Can you work these out from the model? Positions are in its coordinate system, mm. Round coordinates to 2 decimals unless told otherwise and drop trailing zeros. Write each loop counter-clockwise with the first axis right and the second up, starting at its lowest first coordinate (ties: lowest second). Pieces come first, ordered by that corner, then holes. Notation, with made-up numbers: M -18,-27.5 L 41,-27.5 A25 ccw 41,1.5 Z; hole C 66,34 d5. An arc over 180 degrees is marked long. Answer as a JSON object with one key per item and string values. Group by question number.
1) Suppose I cut it at A-A, the plane x = 40. Write out the boundary of the cut face in (y, z), and give its area (3 significant figures).
2) I'm going to push a flat-ended pin straight in: pin 1 Ø3.5 at (x, z) = (60, 0) entering from +Y. Where does the tip first touch, or does it pass through?
3) If we mould it in two halves opening along X, with no side actions, what happens to faces 1 (the flat face through (31, 1, 4)), 2 (the cylindrical face through (8.536, 1.521, -0.325)), 3 (the cylindrical face through (74, 1, 0))? For each: +X half, -X half, draft (parallel to the pull), parting line (faces both ways), or undercut.
4) Please list where these lines run through material, in increasing order: L1, parallel to Z at x = 70, y = 2.2; L2, parallel to Z at x = 10.5, y = 0.6; L3, parallel to X at y = 2.2, z = -3. Write a range as [from, to].
5) Suppose I cut it at B-B, the plane y = 0.8. State how many separate pieces and enclosed holes the cut face has, and give its area (3 significant figures).
from build123d import *

# Parameters (mm, degrees)
OUTER_BODY_DEPTH = 3
SKETCH8_R        = 1.5
HOLES_DEPTH      = 75.168726563


with BuildPart() as part:
    # Sketch1 → Outer Body (new body)
    with BuildSketch(Plane(origin=(0, 0, 0), x_dir=(1, 0, 0), z_dir=(0, 1, 0))):
        with BuildLine():
            Line((-10, 4), (70, 4))
            ThreePointArc((70, 4), (74, 0), (70, -4))
            Line((70, -4), (-10, -4))
            ThreePointArc((-10, -4), (-14, 0), (-10, 4))
        make_face()
    extrude(amount=OUTER_BODY_DEPTH)

    # Sketch8 → Holes (cut, through all)
    with BuildSketch(Plane(origin=(0, 3, 0), x_dir=(1, 0, 0), z_dir=(0, 1, 0))):
        with Locations(Location((-10, 0, 0), (0, 0, 270))):
            Circle(SKETCH8_R)
        with Locations(Location((0, 0, 0), (0, 0, 270))):
            Circle(SKETCH8_R)
        with Locations(Location((50, 0, 0), (0, 0, 270))):
            Circle(SKETCH8_R)
        with Locations(Location((70, 0, 0), (0, 0, 270))):
            Circle(SKETCH8_R)
        with Locations(Location((60, 0, 0), (0, 0, 270))):
            Circle(SKETCH8_R)
        with Locations(Location((10, 0, 0), (0, 0, 270))):
            Circle(SKETCH8_R)
        with Locations(Location((20, 0, 0), (0, 0, 270))):
            Circle(SKETCH8_R)
        with Locations(Location((30, 0, 0), (0, 0, 270))):
            Circle(SKETCH8_R)
        with Locations(Location((40, 0, 0), (0, 0, 270))):
            Circle(SKETCH8_R)
    extrude(amount=-HOLES_DEPTH, mode=Mode.SUBTRACT)


solid = part.part
Results:
{
 "1": {"outline": "M 0,-4 L 3,-4 L 3,-1.5 L 0,-1.5 Z; M 0,1.5 L 3,1.5 L 3,4 L 0,4 Z", "area": "15.0 mm^2"},
 "2": {"pin 1": "y = 3"},
 "3": {"face 1": "draft", "face 2": "undercut", "face 3": "+X half"},
 "4": {"L1": "[-4, -1.5], [1.5, 4]", "L2": "[-4, -1.41], [1.41, 4]", "L3": "[-12.65, 72.65]"},
 "5": {"separate pieces": "1", "enclosed holes": "9", "area": "627 mm^2"}
}
